```python
from build123d import *

# Parameters (mm, degrees)
SKETCH_1_W          = 80
SKETCH_1_H          = 20
EXTRUDE_1_DEPTH     = 10
FILLET_1_R          = 2
EXTRUDE_2_DEPTH     = 5.5
SKETCH_3_W          = 4
SKETCH_3_H          = 5
CUT_EXTRUDE_1_DEPTH = 77.5
SKETCH_4_W          = 3
SKETCH_4_H          = 10
CUT_EXTRUDE_2_DEPTH = 5
FILLET_2_R          = 2


with BuildPart() as part:
    # Эскиз1 → Бобышка-Вытянуть1 (new body)
    with BuildSketch(Plane.XY):
        with Locations((-31.304142693, -21.180034522)):
            Rectangle(SKETCH_1_W, SKETCH_1_H)
    extrude(amount=EXTRUDE_1_DEPTH)

    # Скругление1
    fillet_1_edges = [part.edges().sort_by_distance(p)[0] for p in [
        (-71.304142693, -11.180034522, 5),
        (-71.304142693, -31.180034522, 5),
    ]]
    fillet(fillet_1_edges, radius=FILLET_1_R)

    # Эскиз2 → Бобышка-Вытянуть2 (add)
    with BuildSketch(Plane(origin=(8.695857307, 0, 0), x_dir=(0, 0, -1), z_dir=(1, 0, 0))):
        Polygon((-10, -31.180034522), (-10, -36.180034522), (5, -36.180034522), (5, -6.180034522), (-10, -6.180034522), (-10, -11.180034522), align=None)
    extrude(amount=EXTRUDE_2_DEPTH)

    # Эскиз3 → Вырез-Вытянуть1 (cut)
    with BuildSketch(Plane(origin=(14.195857307, 0, 0), x_dir=(0, 0, -1), z_dir=(1, 0, 0))):
        with Locations((-2, -21.180034522)):
            Rectangle(SKETCH_3_W, SKETCH_3_H)
    extrude(amount=-CUT_EXTRUDE_1_DEPTH, mode=Mode.SUBTRACT)

    # Эскиз4 → Вырез-Вытянуть2 (cut)
    with BuildSketch(Plane(origin=(0, 0, 0), x_dir=(-1, 0, 0), z_dir=(0, 0, -1))):
        with Locations((-3.695857307, -21.180034522)):
            Rectangle(SKETCH_4_W, SKETCH_4_H)
        with Locations((56.304142693, -21.180034522)):
            Rectangle(SKETCH_4_W, SKETCH_4_H)
        with Locations((44.304142693, -21.180034522)):
            Rectangle(SKETCH_4_W, SKETCH_4_H)
        with Locations((32.304142693, -21.180034522)):
            Rectangle(SKETCH_4_W, SKETCH_4_H)
        with Locations((20.304142693, -21.180034522)):
            Rectangle(SKETCH_4_W, SKETCH_4_H)
        with Locations((8.304142693, -21.180034522)):
            Rectangle(SKETCH_4_W, SKETCH_4_H)
    extrude(amount=-CUT_EXTRUDE_2_DEPTH, mode=Mode.SUBTRACT)

    # Скругление2
    fillet_2_edges = [part.edges().sort_by_distance(p)[0] for p in [
        (-63.304142693, -23.680034522, 2),
        (-63.304142693, -21.180034522, 4),
        (-60.554142693, -23.680034522, 4),
        (-63.304142693, -18.680034522, 2),
        (-60.554142693, -18.680034522, 4),
        (-50.304142693, -18.680034522, 4),
        (-38.304142693, -18.680034522, 4),
        (-26.304142693, -18.680034522, 4),
        (-14.304142693, -18.680034522, 4),
        (-2.304142693, -18.680034522, 4),
        (-50.304142693, -23.680034522, 4),
        (-38.304142693, -23.680034522, 4),
        (-26.304142693, -23.680034522, 4),
        (-14.304142693, -23.680034522, 4),
        (-2.304142693, -23.680034522, 4),
    ]]
    fillet(fillet_2_edges, radius=FILLET_2_R)


solid = part.part
```
Here's how the part is built. I have some questions about the finished solid (model axes, mm). A direction names the side the tool comes from. Coordinates: 2 decimals unless noted, no trailing zeros. Loops run counter-clockwise (first coordinate to the right, second up) from the corner with the lowest first, then second, coordinate; pieces in that order, holes last. Notation, with made-up numbers: (-23.5, 85) -> (20.5, 85) arc R7 cw to (20.5, 91) -> close; hole circle Ø7 at (-4, -39). An arc over 180 degrees is marked (long way). Return JSON: item names as keys, results as strings.
1) For faces 1 (the face through (-56, -16.18, 2)), 2 (the face through (-31, -31.18, 5)), 3 (the face through (-26.37, -23.11, 3.4)), which set-ups out of +Z, -Z, +X, -X, +Y, -Y let a thin tool reach every point of the face, with its end or its side?
Results below:
{"face 1": "-Z", "face 2": "+Z, -Z, -X, -Y", "face 3": "-Z, +X"}
2) Thinking about a two-plate mould opening in Z: for faces 4 (the face through (10, -23.68, 2)), 5 (the face through (4, -16.18, 2)), 6 (the face through (10, -18.68, 2)), 7 (the face through (-41, -17, 0)), which applies, +Z half, -Z half, draft (parallel to the pull), parting line (faces both ways), or undercut?
Results below:
{"face 4": "undercut", "face 5": "draft", "face 6": "undercut", "face 7": "-Z half"}
3) If we section it at C-C, the plane z = -1.5: Write out the boundary of the cut face in (x, y).
Results below:
{"outline": "(8.7, -36.18) -> (14.2, -36.18) -> (14.2, -6.18) -> (8.7, -6.18) -> close"}
4) Will these pins go through, and if not, where does the flat tip stop? pin 1 (1 mm diameter, centred on x = -13.5, z = 0.5, fed in from +Y); pin 2 (0.8 mm diameter, centred on x = -59.5, y = -21, fed in from -Z); pin 3 (1 mm diameter, centred on x = -37.5, z = 0.5, fed in from -Y).
Results below:
{"pin 1": "y = -11.18", "pin 2": "z = 4", "pin 3": "y = -31.18"}
5) I need wall thicknesses on line 1 (Y direction, x = 6, z = 0.5); line 2 (Y direction, x = 4.5, z = 6.75); line 3 (Z direction, x = -64.5, y = -15). Which ranges of each line are inside material? Lowest first, please. Write a range as from..to.
Results below:
{"line 1": "-31.18..-23.68, -18.68..-11.18", "line 2": "-31.18..-11.18", "line 3": "0..10"}
6) If we section it at D-D, the plane x = -20: Write out the boundary of the cut face in (y, z), then the cut area to 3 significant figures.
Results below:
{"outline": "(-31.18, 0) -> (-26.18, 0) -> (-26.18, 5) -> (-16.18, 5) -> (-16.18, 0) -> (-11.18, 0) -> (-11.18, 10) -> (-31.18, 10) -> close", "area": "150 mm²"}
7) If we section it at A-A, the plane x = -59.5: Write out the boundary of the cut face in (y, z), then the cut area to 3 significant figures.
Results below:
{"outline": "(-31.18, 0) -> (-23.68, 0) -> (-23.68, 2) arc R2 cw to (-21.68, 4) -> (-20.68, 4) arc R2 cw to (-18.68, 2) -> (-18.68, 0) -> (-11.18, 0) -> (-11.18, 10) -> (-31.18, 10) -> close", "area": "182 mm²"}
